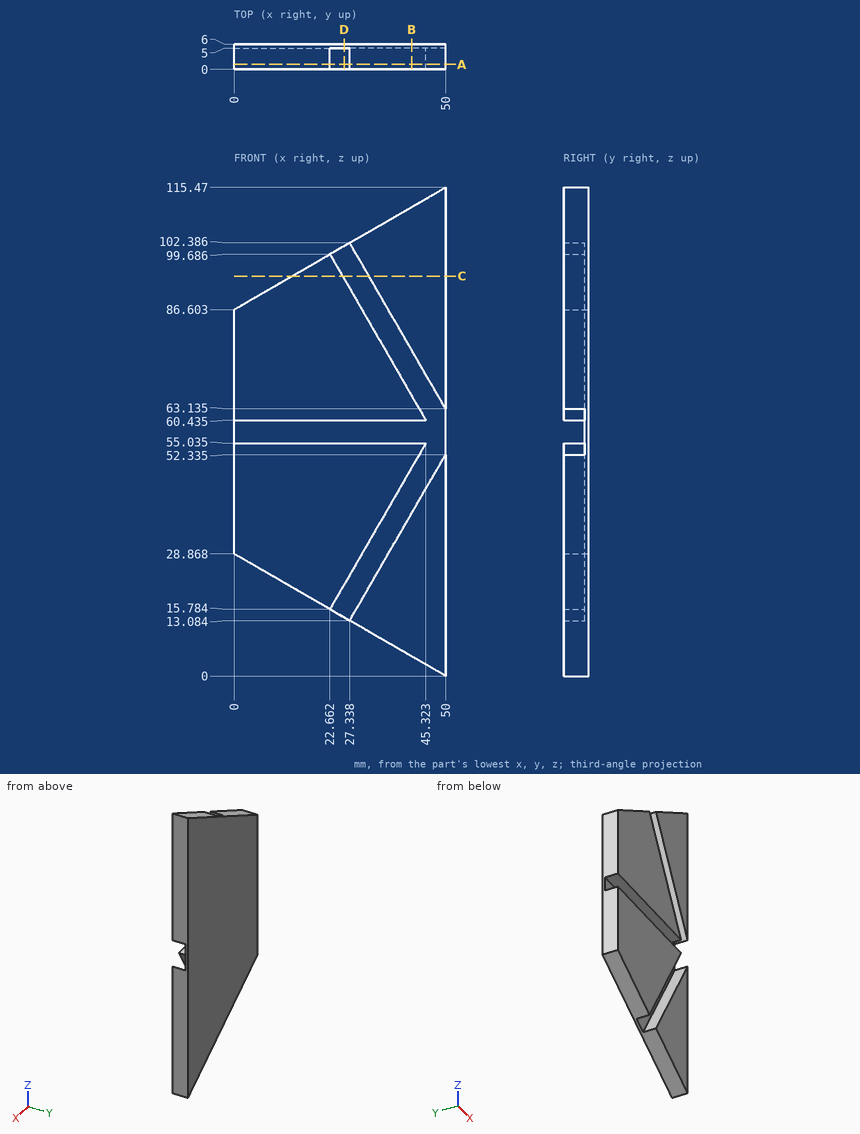
The figure shows three views and two pictorial views of one solid part (mm, origin at its lowest corner). Answer the questions. Coordinates: 2 decimals unless noted, no trailing zeros. Write each loop counter-clockwise with the first axis right and the second up, starting at its lowest first coordinate (ties: lowest second). Pieces come first, ordered by that corner, then holes. Notation, with made-up numbers: (68, 87) -> (73, 87) arc R11 cw to (73, 91) -> close; hole circle Ø5 at (-10.75, 64). An arc over 180 degrees is marked (long way). Return JSON: item names as keys, results as strings.
(1) The part is cut by section D-D on x = 26. Give the vertices of the cut face in (y, z) (1 decimal).
Answers below:
{"outline": "(0, 21.6) -> (5, 21.6) -> (5, 13.9) -> (6, 13.9) -> (6, 101.6) -> (5, 101.6) -> (5, 93.9) -> (0, 93.9) -> (0, 60.4) -> (5, 60.4) -> (5, 55) -> (0, 55) -> close"}
(2) The part is cut by section B-B on x = 42. Give the vertices of the cut face in (y, z) (1 decimal).
Answers below:
{"outline": "(0, 4.6) -> (6, 4.6) -> (6, 110.9) -> (0, 110.9) -> (0, 77) -> (5, 77) -> (5, 66.2) -> (0, 66.2) -> (0, 60.4) -> (5, 60.4) -> (5, 55) -> (0, 55) -> (0, 49.3) -> (5, 49.3) -> (5, 38.5) -> (0, 38.5) -> close"}
(3) The part is cut by section C-C on z = 94.5. Give the vertices of the cut face in (x, y), then the cut area to 3 significant figures.
Answers below:
{"outline": "(13.68, 0) -> (25.66, 0) -> (25.66, 5) -> (31.89, 5) -> (31.89, 0) -> (50, 0) -> (50, 6) -> (13.68, 6) -> close", "area": "187 mm^2"}
(4) The part is cut by section A-A on y = 1.2. Give the vertices of the cut face in (x, z) (1 decimal), then the cut area to 3 significant figures.
Answers below:
{"outline": "(0, 28.9) -> (22.7, 15.8) -> (45.3, 55) -> (0, 55) -> close; (0, 60.4) -> (45.3, 60.4) -> (22.7, 99.7) -> (0, 86.6) -> close; (27.3, 13.1) -> (50, 0) -> (50, 52.3) -> close; (27.3, 102.4) -> (50, 63.1) -> (50, 115.5) -> close", "area": "3,560 mm^2"}
(5) Consider line 1 along Z through (x, y) = (45, 3.05) (1 decimal); line 2 along Z through (x, y) = (27.5, 3.5) (1 decimal); line 3 along Z through (x, y) = (13, 4.95) (1 decimal). Determine where each line is inside the solid, lowest interval first. Write a range as from..to.
Answers below:
{"line 1": "2.9..43.7, 54.5..55, 60.4..61, 71.8..112.6", "line 2": "13..13.4, 24.2..55, 60.4..91.3, 102.1..102.5", "line 3": "21.4..55, 60.4..94.1"}
(6) Each of these flat-tipped pins is pushed along its axis until it touches: P1, Ø3, axis at x = 23, y = 3, coming from the +Z side; P2, Ø1.5, axis at x = 22.5, y = 4.5, coming from the +Z side (1 decimal); P3, Ø3, axis at x = 30.5, y = 1.5, coming from the +Z side. Where does it stop, or does it pass through?
Answers below:
{"P1": "z = 99.69", "P2": "z = 99.9", "P3": "z = 105.08"}
